```python
from build123d import *

# Parameters (mm, degrees)
SKETCH_R     = 4
PAD_DEPTH    = 420
PAD001_DEPTH = 12


with BuildPart() as part:
    # Sketch → Pad (new body)
    with BuildSketch(Plane.YZ):
        Circle(SKETCH_R)
    extrude(amount=PAD_DEPTH)

    # Sketch001 (on Face2 of Pad) → Pad001 (join)
    with BuildSketch(Plane(origin=(0, 0, 0), x_dir=(0, -1, 0), z_dir=(-1, 0, 0))):
        Polygon((7, 4.041452), (0, 8.082904), (-7, 4.041452), (-7, -4.041452), (0, -8.082904), (7, -4.041452), align=None)
    extrude(amount=PAD001_DEPTH)


solid = part.part
```
Input: part model. Units: mm. Frame: model coordinates. A direction names the side the tool comes from. Give positions to 0.01 mm unless a question says otherwise; leave off trailing zeros. Order: outer loops, then holes, each group sorted by start corner. A loop starts at its lowest first (then second) coordinate and runs counter-clockwise, first axis right, second up. Notation, with made-up numbers: M 62,-39 L 74,-39 A9 ccw 74,-26 Z; hole C 27,0.5 d2. An arc over 180 degrees is marked long. Return JSON: item names as keys, results as strings.
Item 1: Ray query, probe 1 along X at (y, z) = (0.25, 4.5); probe 2 along Y at (x, z) = (40, -0.5); probe 3 along Z at (x, y) = (275, 0.75). Return the intervals inside material, ascending.
Solutions:
{"probe 1": "-12 to 0", "probe 2": "-3.97 to 3.97", "probe 3": "-3.93 to 3.93"}
Item 2: First-contact query: P1, Ø5, axis at x = 346, z = -5, coming from the -Y side; P2, Ø3, axis at x = 291.5, y = 1, coming from the +Z side; P3, Ø1, axis at x = 160, z = -5, coming from the +Y side. Flat tips, straight axial feed; report the tip coordinate or a pass-through.
Solutions:
{"P1": "y = -3.12", "P2": "z = 4", "P3": "through"}
Item 3: Cut plane B-B (x = 70). Return loops of the section in (y, z), then the cut area to 3 significant figures.
Solutions:
{"outline": "C 0,0 d8", "area": "50.3 mm^2"}
Item 4: Cut plane A-A (z = 0). Return loops of the section in (x, y).
Solutions:
{"outline": "M -12,-7 L 0,-7 L 0,-4 L 420,-4 L 420,4 L 0,4 L 0,7 L -12,7 Z"}
Item 5: Access query for faces 1 (the cylindrical face through (207.06, -0.867, -3.905)), 2 (the flat face through (-6, -7, 0)). Directions: +Z, -Z, +X, -X, +Y, -Y. A direction counts if a zero-diameter tool reaches every point of the face in a straight line with its end or side. Return the directions, or none.
Solutions:
{"face 1": "+X", "face 2": "+Z, -Z, +X, -X, -Y"}
